Can you work these out from the model? Positions are in its coordinate system, mm. A direction names the side the tool comes from. Round coordinates to 2 decimals unless told otherwise and drop trailing zeros. Write each loop counter-clockwise with the first axis right and the second up, starting at its lowest first coordinate (ties: lowest second). Pieces come first, ordered by that corner, then holes. Notation, with made-up numbers: M 39,82 L 62,82 A15 ccw 62,103 Z; hole C 46.5,35.25 d4. An arc over 180 degrees is marked long. Answer as a JSON object with one key per item and string values. Group by question number.
1) Suppose I cut it at B-B, the plane z = 0. Write out the boundary of the cut face in (x, y), and give its area (3 significant figures).
2) If we mould it in two halves opening along Z, with no side actions, what happens to faces 1 (the cylindrical face through (0.248, 2.218, -5.645)), 2 (the flat face through (6, 1, 1.5)), 3 (the cylindrical face through (-4.503, 2.218, -5.872)), 4 (the flat face through (-1, 0, -6))? For each: +Z half, -Z half, draft (parallel to the pull), parting line (faces both ways), or undercut.
3) Suppose I cut it at C-C, the plane y = 4.1. Write out the boundary of the cut face in (x, z), and give its area (3 significant figures).
4) On a 3-axis mill with a long thin cutter (end or side, diameter ignored), from which of +Z, -Z, +X, -X, +Y, -Y can I reach the whole of each face in a straight line? I mean faces 5 (the flat face through (6, 1, -1.5)), 6 (the flat face through (-4, 5, -5)). Say none if no direction works.
5) Suppose I cut it at A-A, the plane x = 0. Write out the boundary of the cut face in (y, z), and give its area (3 significant figures).
6) Please list where these lines run through material, in increasing order: L1, parallel to X at y = 2.8, z = 0; L2, parallel to X at y = 3.95, z = 1.5; L3, parallel to Z at x = 4, y = 4. Write a range as [from, to].
7) I'm going to push flat-ended pins straight in: pin 1 Ø1.5 at (x, y) = (-0.5, 1) entering from -Z; pin 2 Ø5 at (x, z) = (-2, -2.5) entering from +Y; pin 3 Ø0.6 at (x, z) = (-6, -0.5) entering from -Y; pin 4 Ø0.8 at (x, y) = (6.5, 0.5) entering from +Z. Where does each tip first touch, or does it pass through?
from build123d import *

# Parameters (mm, degrees)
SKETCH1_R           = 7.4
SKETCH1_R_2         = 5.65
BOSS_EXTRUDE1_DEPTH = 5
SKETCH2_W           = 27.497480526
SKETCH2_H           = 3
CUT_EXTRUDE2_DEPTH  = 1.6
FILLET1_R           = 0.5
CHAMFER1_SIZE       = 0.5


with BuildPart() as part:
    # Sketch1 → Boss-Extrude1 (new body)
    with BuildSketch(Plane(origin=(0, 0, 0), x_dir=(1, 0, 0), z_dir=(0, 1, 0))):
        with Locations(Location((0, 0, 0), (0, 0, 270))):
            Circle(SKETCH1_R)
        with Locations(Location((0, 0, 0), (0, 0, 270))):
            Circle(SKETCH1_R_2, mode=Mode.SUBTRACT)
    extrude(amount=BOSS_EXTRUDE1_DEPTH)

    # Sketch2 → Cut-Extrude2 (cut)
    with BuildSketch(Plane(origin=(0, 0, 0), x_dir=(1, 0, 0), z_dir=(0, 1, 0))):
        Rectangle(SKETCH2_W, SKETCH2_H)
    extrude(amount=CUT_EXTRUDE2_DEPTH, mode=Mode.SUBTRACT)

    # Fillet1
    fillet1_edges = [part.edges().sort_by_distance(p)[0] for p in [
        (-3.423996203, 0, 4.494301948),
        (4.672258554, 0, 5.738466694),
        (0, 5, -7.4),
    ]]
    fillet(fillet1_edges, radius=FILLET1_R)

    # Chamfer1
    chamfer1_edges = [part.edges().sort_by_distance(p)[0] for p in [
        (0, 5, -5.65),
    ]]
    chamfer(chamfer1_edges, length=CHAMFER1_SIZE)


solid = part.part
Results:
{
 "1": {"outline": "M -7.4,1.6 L -5.65,1.6 L -5.65,4.5 L -6.15,5 L -6.9,5 A0.5 ccw -7.4,4.5 Z; M 5.65,1.6 L 7.4,1.6 L 7.4,4.5 A0.5 ccw 6.9,5 L 6.15,5 L 5.65,4.5 Z", "area": "11.5 mm^2"},
 "2": {"face 1": "undercut", "face 2": "undercut", "face 3": "parting line", "face 4": "draft"},
 "3": {"outline": "C 0,0 d14.8; hole C 0,0 d11.3", "area": "71.7 mm^2"},
 "4": {"face 5": "+X, -X, -Y", "face 6": "+Z, -Z, +X, -X, +Y"},
 "5": {"outline": "M 0,-7.4 L 4.5,-7.4 A0.5 ccw 5,-6.9 L 5,-6.15 L 4.5,-5.65 L 0,-5.65 Z; M 0,6.15 A0.5 ccw 0.5,5.65 L 4.5,5.65 L 5,6.15 L 5,6.9 A0.5 ccw 4.5,7.4 L 0.5,7.4 A0.5 ccw 0,6.9 Z", "area": "17.0 mm^2"},
 "6": {"L1": "[-7.4, -5.65], [5.65, 7.4]", "L2": "[-7.25, -5.45], [5.45, 7.25]", "L3": "[-6.23, -3.99], [3.99, 6.23]"},
 "7": {"pin 1": "z = -7.4", "pin 2": "y = 4.55", "pin 3": "y = 1.6", "pin 4": "z = 4.19"}
}
